Work out the finished part from the listing and answer in its coordinate system (mm). A direction names the side the tool comes from. Give positions to 0.01 mm unless a question says otherwise; leave off trailing zeros. Order: outer loops, then holes, each group sorted by start corner. A loop starts at its lowest first (then second) coordinate and runs counter-clockwise, first axis right, second up.
```python
from build123d import *

# Parameters (mm, degrees)
SKETCH1_R           = 5
SKETCH1_W           = 100
SKETCH1_H           = 270
BOSS_EXTRUDE1_DEPTH = 30
FILLET1_R           = 10


with BuildPart() as part:
    # Sketch1 → Boss-Extrude1 (new body)
    with BuildSketch(Plane.XY):
        with BuildLine():
            Line((0, 0), (150, 0))
            Line((150, 0), (150, 330))
            ThreePointArc((150, 330), (75, 405), (0, 330))
            Line((0, 330), (0, 0))
        make_face()
        with Locations((75, 330)):
            Circle(SKETCH1_R, mode=Mode.SUBTRACT)
        with Locations((75, 160)):
            Rectangle(SKETCH1_W, SKETCH1_H, mode=Mode.SUBTRACT)
    extrude(amount=BOSS_EXTRUDE1_DEPTH)

    # Fillet1
    fillet1_edges = [part.edges().sort_by_distance(p)[0] for p in [
        (125, 295, 15),
        (25, 295, 15),
        (25, 25, 15),
        (125, 25, 15),
    ]]
    fillet(fillet1_edges, radius=FILLET1_R)


solid = part.part
```
1. Which of the six approach directions +Z, -Z, +X, -X, +Y, -Y give full straight-line access (tool end or side, diameter ignored) to faces 1 (the face through (74, 295, 15)), 2 (the face through (24, 250, 30))?
Findings below:
face 1: +Z, -Z
face 2: +Z, +X, -X, +Y, -Y
2. Given P1, Ø1.5, axis at x = 116, z = 18.5, coming from the +Y side; P2, Ø8, axis at x = 75, y = 330, coming from the +Z side; P3, Ø1.5, axis at x = 129.5, z = 12, coming from the +Y side; P4, Ø9, axis at x = 67.5, z = 16.5, coming from the +Y side, each flat-ended and moving along its own axis, determine where each tip first touches the part or whether it passes through.
Findings below:
P1: stops at y = 393.28
P2: passes through
P3: stops at y = 382.31
P4: stops at y = 404.94
3. The part is cut by section D-D (x = 56). Write down the section's boundary in (y, z), then the cut area to 3 significant figures.
Findings below:
outline: (0, 0) - (25, 0) - (25, 30) - (0, 30) - close; (295, 0) - (402.55, 0) - (402.55, 30) - (295, 30) - close
area: 3,980 mm2
4. The mould has two halves that part along Y. Classify faces 3 (the face through (150, 163, 15)), 4 (the face through (74, 0, 15)), 5 (the face through (76.65, 404.98, 14.79)), 6 (the face through (74.349, 334.957, 14.79)): pulls with the +Y half, pulls with the -Y half, needs draft (parallel to the pull), parting line crosses it, or undercut.
Findings below:
face 3: needs draft
face 4: pulls with the -Y half
face 5: pulls with the +Y half
face 6: undercut
5. The part is cut by section C-C (x = 75). Write down the section's boundary in (y, z).
Findings below:
outline: (0, 0) - (25, 0) - (25, 30) - (0, 30) - close; (295, 0) - (325, 0) - (325, 30) - (295, 30) - close; (335, 0) - (405, 0) - (405, 30) - (335, 30) - close
6. The part is cut by section B-B (y = 225.5). Write down the section's boundary in (x, z), then the cut area to 3 significant figures.
Findings below:
outline: (0, 0) - (25, 0) - (25, 30) - (0, 30) - close; (125, 0) - (150, 0) - (150, 30) - (125, 30) - close
area: 1,500 mm2
7. Straight lines are drawn through the part: probe 1 along Y at (x, z) = (75, 20.5); probe 2 along X at (y, z) = (330, 18.25); probe 3 along X at (y, z) = (249, 11.25). For each, find the intervals that lie inside material, in ascending order.
Findings below:
probe 1: y = 0 to 25, 295 to 325, 335 to 405
probe 2: x = 0 to 70, 80 to 150
probe 3: x = 0 to 25, 125 to 150
8. The part is cut by section A-A (z = 11.75). Write down the section's boundary in (x, y), then the cut area to 3 significant figures.
Findings below:
outline: (0, 0) - (150, 0) - (150, 330) arc R75 ccw to (0, 330) - close; hole (25, 35) arc R10 ccw to (35, 25) - (115, 25) arc R10 ccw to (125, 35) - (125, 285) arc R10 ccw to (115, 295) - (35, 295) arc R10 ccw to (25, 285) - close; hole circle Ø10 at (75, 330)
area: 31,300 mm2
